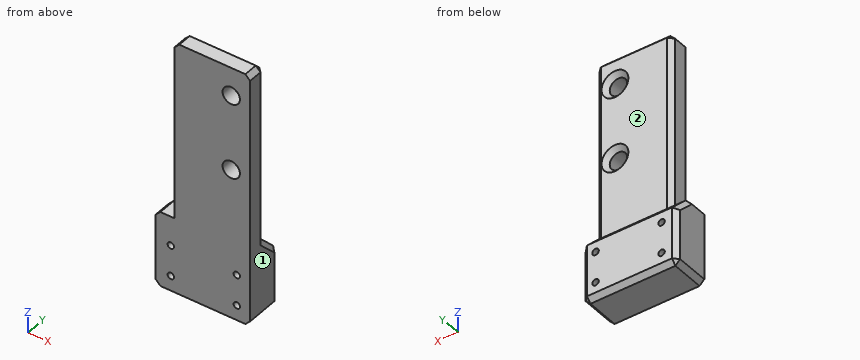
```python
from build123d import *

# Parameters (mm, degrees)
SKETCH1_W           = 31.75
SKETCH1_H           = 85.725
SKETCH1_R           = 2.921
BOSS_EXTRUDE1_DEPTH = 12.7
SKETCH2_W           = 60.325
SKETCH2_H           = 6.35
CUT_EXTRUDE1_DEPTH  = 93.293705771
SKETCH3_R           = 1.0922
SKETCH3_W           = 6.35
SKETCH3_H           = 60.325
CUT_EXTRUDE2_DEPTH  = 93.293705771
CHAMFER1_SIZE       = 6.35
CHAMFER2_SIZE       = 1.5875


with BuildPart() as part:
    # Sketch1 → Boss-Extrude1 (new body)
    with BuildSketch(Plane(origin=(0, 0, 0), x_dir=(1, 0, 0), z_dir=(0, 1, 0))):
        with Locations((15.875, 42.8625)):
            Rectangle(SKETCH1_W, SKETCH1_H)
        with Locations(Location((25.4, 9.525, 0), (0, 0, 270))):
            Circle(SKETCH1_R, mode=Mode.SUBTRACT)
        with Locations(Location((25.4, 34.925, 0), (0, 0, 270))):
            Circle(SKETCH1_R, mode=Mode.SUBTRACT)
    extrude(amount=BOSS_EXTRUDE1_DEPTH)

    # Sketch2 → Cut-Extrude1 (cut, through all)
    with BuildSketch(Plane(origin=(31.75, 0, 0), x_dir=(0, 0, -1), z_dir=(1, 0, 0))):
        with Locations((30.1625, 9.525)):
            Rectangle(SKETCH2_W, SKETCH2_H)
    extrude(amount=-CUT_EXTRUDE1_DEPTH, mode=Mode.SUBTRACT)

    # Sketch3 → Cut-Extrude2 (cut, through all)
    with BuildSketch(Plane.XZ):
        with Locations(Location((27.2796, -70.231, 0), (0, 0, 270))):
            Circle(SKETCH3_R)
        with Locations(Location((5.08, -80.645, 0), (0, 0, 270))):
            Circle(SKETCH3_R)
        with Locations(Location((27.2796, -80.645, 0), (0, 0, 270))):
            Circle(SKETCH3_R)
        with Locations(Location((5.08, -70.231, 0), (0, 0, 270))):
            Circle(SKETCH3_R)
        with Locations((3.175, -30.1625)):
            Rectangle(SKETCH3_W, SKETCH3_H)
    extrude(amount=-CUT_EXTRUDE2_DEPTH, mode=Mode.SUBTRACT)

    # Chamfer1
    chamfer1_edges = [part.edges().sort_by_distance(p)[0] for p in [
        (15.875, 12.7, -60.325),
    ]]
    chamfer(chamfer1_edges, length=CHAMFER1_SIZE)

    # Chamfer2
    chamfer2_edges = [part.edges().sort_by_distance(p)[0] for p in [
        (15.875, 12.7, -85.725),
        (31.75, 3.175, 0),
        (25.4, 6.35, -12.446),
        (25.4, 6.35, -37.846),
        (0, 3.175, -60.325),
        (31.75, 6.35, -30.1625),
        (19.05, 6.35, 0),
        (6.35, 6.35, -30.1625),
        (0, 12.7, -76.2),
        (6.35, 3.175, 0),
        (0, 6.35, -85.725),
        (31.75, 6.35, -85.725),
        (31.75, 12.7, -76.2),
        (31.75, 9.525, -63.5),
        (0, 9.525, -63.5),
    ]]
    chamfer(chamfer2_edges, length=CHAMFER2_SIZE)


solid = part.part
```
Geometry check sheet. Reference: the model listing, model coordinates, mm. Face numbers are marked on the shaded views. A direction names the side the tool comes from. Coordinates: 2 decimals unless noted, no trailing zeros. Loops run counter-clockwise (first coordinate to the right, second up) from the corner with the lowest first, then second, coordinate; pieces in that order, holes last. Notation, with made-up numbers: (79.25, -37) - (123.25, -37) arc R24 cw to (123.25, -4) - close; hole circle Ø5 at (-26.75, -23.5). An arc over 180 degrees is marked (long way). One line per item, written item: value. Start each with the question number.
(1) Cross-section at B-B on z = -40.5. Enter the section's corners in (x, y), plus the area to 3 significant figures.
(2) Material ranges on line 1 (Z direction, x = 25.4, y = 1.7) (3 decimals); line 2 (Z direction, x = 4.5, y = 1.5) (3 decimals); line 3 (Z direction, x = 3, y = 6) (3 decimals), recorded low to high. Write a range as [from, to].
(3) Cross-section at A-A on x = 25.4. Count the separate pieces of the cut face and the enclosed holes in it, plus the area to 3 significant figures.
(4) Tool access check on the marked faces 1 and 2. Record the directions out of +Z, -Z, +X, -X, +Y, -Y that give a thin tool (end or side, any length) a straight path to the whole face; none if there is none.
(5) Depth check by flat-ended pin: P1, Ø4, axis at y = 1.5, z = -21, coming from the -X side; P2, Ø3, axis at x = 27.28, z = -80.64, coming from the -Y side; P3, Ø1, axis at y = 5.5, z = -15, coming from the -X side; P4, Ø18, axis at x = 22, z = -39, coming from the +Y side. Enter the tip coordinate at first touch or a pass-through.
Results below:
1. outline: (6.35, 0) - (31.75, 0) - (31.75, 4.76) - (30.16, 6.35) - (7.94, 6.35) - (6.35, 4.76) - close
1. area: 159 mm2
2. line 1: z = [-85.725, -37.846], [-32.004, -12.446], [-6.604, 0]
2. line 2: z = [-85.725, -81.57], [-79.72, -71.156], [-69.306, -60.325]
2. line 3: z = [-85.725, -60.325]
3. separate pieces: 3
3. enclosed holes: 0
3. area: 604 mm2
4. face 1: +Z, -Z, +X, +Y, -Y
4. face 2: +Z, +X, -X, +Y
5. P1: stops at x = 6.35
5. P2: stops at y = 0
5. P3: stops at x = 6.59
5. P4: stops at y = 6.35
